from build123d import *

# Parameters (mm, degrees)
F0_R      = 16
F0_R_2    = 14.5
F1_DEPTH  = 55
F2_R      = 16
F3_DEPTH  = 2
F4_R      = 16
F5_DEPTH  = 2
F7_DEPTH  = 59.001
F9_DEPTH  = 58
F10_W     = 23
F10_H     = 55
F11_DEPTH = 3
F13_DEPTH = 11.3


with BuildPart() as f1:
    # F0 (on Top) → F1 (new body)
    with BuildSketch(Plane.XY):
        Circle(F0_R)
        Circle(F0_R_2, mode=Mode.SUBTRACT)
    extrude(amount=F1_DEPTH)

    # F2 (on face) → F3 (join)
    with BuildSketch(Plane.XY.offset(55)):
        Circle(F2_R)
    extrude(amount=F3_DEPTH)

    # F4 (on face) → F5 (join)
    with BuildSketch(Plane(origin=(0, 0, 0), x_dir=(1, 0, 0), z_dir=(0, 0, -1))):
        Circle(F4_R)
    extrude(amount=F5_DEPTH)

    # F6 (on face) → F7 (cut, through all)
    with BuildSketch(Plane(origin=(0, 0, -2), x_dir=(1, 0, 0), z_dir=(0, 0, -1))):
        with BuildLine():
            Line((-11.5, 11.1242977306), (11.5, 11.1242977306))
            ThreePointArc((11.5, 11.1242977306), (0, 16), (-11.5, 11.1242977306))
        make_face()
    extrude(amount=-F7_DEPTH, mode=Mode.SUBTRACT)

    # F8 (on face) → F9 (join)
    with BuildSketch(Plane(origin=(0, 0, -2), x_dir=(1, 0, 0), z_dir=(0, 0, -1))):
        with BuildLine():
            Line((-11.5, -11.1242977306), (-11.5, 11.1242977306))
            ThreePointArc((-11.5, 11.1242977306), (-16, 0), (-11.5, -11.1242977306))
        make_face()
        with BuildLine():
            ThreePointArc((-11.5, -11.1242977306), (0, -16), (11.5, -11.1242977306))
            Line((11.5, -11.1242977306), (-11.5, -11.1242977306))
        make_face()
        with BuildLine():
            ThreePointArc((11.5, -11.1242977306), (16, 0), (11.5, 11.1242977306))
            Line((11.5, 11.1242977306), (11.5, -11.1242977306))
        make_face()
    extrude(amount=-F9_DEPTH)

    # F10 (on face) → F11 (cut)
    with BuildSketch(Plane.XZ.offset(11.1242977306)):
        with Locations((0, 27.5)):
            Rectangle(F10_W, F10_H)
    extrude(amount=-F11_DEPTH, mode=Mode.SUBTRACT)

    # F12 (on face) → F13 (join)
    with BuildSketch(Plane(origin=(0, 0, 55), x_dir=(1, 0, 0), z_dir=(0, 0, -1))):
        with BuildLine():
            Line((11.5, -8.8317608663), (11.5, 11.1242977306))
            Line((11.5, 11.1242977306), (-11.5, 11.1242977306))
            Line((-11.5, 11.1242977306), (-11.5, -8.8317608663))
            ThreePointArc((-11.5, -8.8317608663), (-10.4632462758, -10.0384499487), (-9.3005376189, -11.1242977306))
            Line((-9.3005376189, -11.1242977306), (9.3005376189, -11.1242977306))
            ThreePointArc((9.3005376189, -11.1242977306), (10.4632462758, -10.0384499487), (11.5, -8.8317608663))
        make_face()
        with BuildLine():
            Line((0.65, -4.4), (-0.65, -4.4))
            ThreePointArc((-0.65, -4.4), (-8.0759144982, -7.4759144982), (-5, -0.05))
            Line((-5, -0.05), (-5, 0.05))
            ThreePointArc((-5, 0.05), (-8.0759144982, 7.4759144982), (-0.65, 4.4))
            Line((-0.65, 4.4), (0.65, 4.4))
            ThreePointArc((0.65, 4.4), (5, 8.75), (9.35, 4.4))
            ThreePointArc((9.35, 4.4), (8.0759144982, 1.3240855018), (5, 0.05))
            Line((5, 0.05), (5, -0.05))
            ThreePointArc((5, -0.05), (8.0759144982, -1.3240855018), (9.35, -4.4))
            ThreePointArc((9.35, -4.4), (5, -8.75), (0.65, -4.4))
        make_face(mode=Mode.SUBTRACT)
        with BuildLine():
            ThreePointArc((-5, -0.05), (-1.9240855018, -1.3240855018), (-0.65, -4.4))
            Line((-0.65, -4.4), (0.65, -4.4))
            ThreePointArc((0.65, -4.4), (1.9240855018, -1.3240855018), (5, -0.05))
            Line((5, -0.05), (5, 0.05))
            ThreePointArc((5, 0.05), (1.9240855018, 1.3240855018), (0.65, 4.4))
            Line((0.65, 4.4), (-0.65, 4.4))
            ThreePointArc((-0.65, 4.4), (-1.9240855018, 1.3240855018), (-5, 0.05))
            Line((-5, 0.05), (-5, -0.05))
        make_face()
    extrude(amount=F13_DEPTH)


solid = f1.part
Source: CAD feature listing. Evaluate the final solid. Frame: model axes, mm. A direction names the side the tool comes from. Give positions to 0.01 mm unless a question says otherwise; leave off trailing zeros. Write each loop counter-clockwise with the first axis right and the second up, starting at its lowest first coordinate (ties: lowest second). Pieces come first, ordered by that corner, then holes. Notation, with made-up numbers: M 55,67.25 L 109,67.25 A28 ccw 109,90.25 Z; hole C 81,64.5 d4. An arc over 180 degrees is marked long. Return JSON: item names as keys, results as strings. Group by question number.
1) Cut plane A-A, the plane z = 44.5. Output: boundary loops of the cut face in (x, y).
2) Pin query (flat end, axial travel): P1, Ø15, axis at x = -3, z = 30.5, coming from the -Y side; P2, Ø2, axis at y = 13, z = 46.5, coming from the -X side; P3, Ø1.5, axis at x = 1.5, z = 6.5, coming from the +Y side. Return the tip coordinate at first contact, or that it passes through.
3) Cut plane D-D, the plane x = 0. Output: boundary loops of the cut face in (y, z).
4) Pull-direction query (Z, two-part tool) for faces 1 (the face through (0, -11.124, 50)), 2 (the face through (0, 3, 57)), 3 (the face through (-5, 4, 55)); classes: pulls with the +Z half, pulls with the -Z half, needs draft (parallel to the pull), parting line crosses it, or undercut.
5) Set-up query: faces 4 (the face through (11.5, -1, 22)), 5 (the face through (5, -4, 55)), 6 (the face through (0, 2, -2)). Return all of +Z, -Z, +X, -X, +Y, -Y with unobstructed straight access to the full face (end or side cutting, diameter ignored); none if empty.
6) Cut plane C-C, the plane z = 11. Output: boundary loops of the cut face in (x, y), plus the area to 3 significant figures.
7) Cut plane B-B, the plane y = 2. Output: boundary loops of the cut face in (x, z).
8) Material intervals for line 1 along Z through (x, y) = (11, -10); line 2 along Z through (x, y) = (-6, 4.5); line 3 along X through (y, z) = (0, 38), sorted ascending. Write a range as [from, to].
Recorded:
{
 "1": {"outline": "M -11.5,-11.12 L 11.5,-11.12 A16 ccw long Z; hole C -5,-4.4 d8.7; hole C -5,4.4 d8.7; hole C 5,-4.4 d8.7; hole C 5,4.4 d8.7"},
 "2": {"P1": "stops at y = 10", "P2": "stops at x = -10.58", "P3": "stops at y = 15.98"},
 "3": {"outline": "M -11.12,-2 L 16,-2 L 16,57 L -11.12,57 L -11.12,43.7 L 11.12,43.7 L 11.12,0 L -11.12,0 Z"},
 "4": {"face 1": "needs draft", "face 2": "pulls with the +Z half", "face 3": "undercut"},
 "5": {"face 4": "-Y", "face 5": "none", "face 6": "-Z, +X, -X, +Y, -Y"},
 "6": {"outline": "M -11.5,-11.12 L -11.5,8.83 A14.5 cw -9.3,11.12 L 9.3,11.12 A14.5 cw 11.5,8.83 L 11.5,-11.12 A16 ccw long Z", "area": "220 mm²"},
 "7": {"outline": "M -15.87,-2 L 15.87,-2 L 15.87,57 L -15.87,57 Z; hole M -11.5,0 L 11.5,0 L 11.5,43.7 L 8.63,43.7 L 8.63,55 L 1.37,55 L 1.37,43.7 L -1.37,43.7 L -1.37,55 L -8.63,55 L -8.63,43.7 L -11.5,43.7 Z"},
 "8": {"line 1": "z = [-2, 0], [43.7, 57]", "line 2": "z = [-2, 0], [55, 57]", "line 3": "x = [-16, -11.5], [11.5, 16]"}
}
